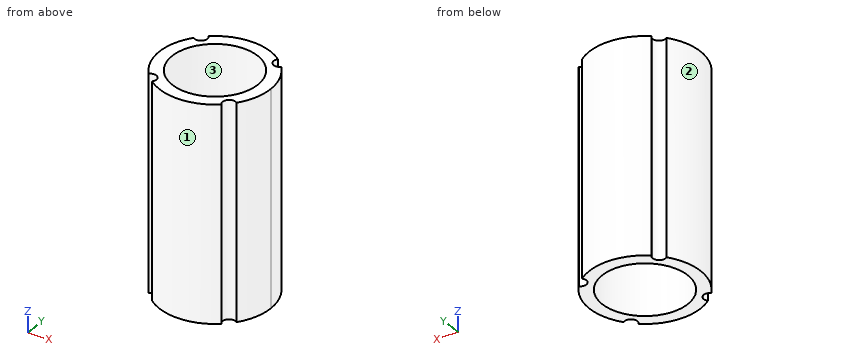
```python
from build123d import *

# Parameters (mm, degrees)
F0_R     = 12.7
F1_DEPTH = 63.5


with BuildPart() as f1:
    # F0 (on Top) → F1 (new body)
    with BuildSketch(Plane.XY):
        with BuildLine():
            ThreePointArc((12.941414, -10.251824), (15.592351, -5.427585), (16.51, 0))
            ThreePointArc((16.51, 0), (15.592351, 5.427585), (12.941414, 10.251824))
            ThreePointArc((12.941414, 10.251824), (10.327295, 10.327295), (10.251824, 12.941414))
            ThreePointArc((10.251824, 12.941414), (0, 16.51), (-10.251824, 12.941414))
            ThreePointArc((-10.251824, 12.941414), (-9.894038, 12.352251), (-9.769333, 11.674333))
            ThreePointArc((-9.769333, 11.674333), (-10.894835, 9.936113), (-12.941414, 10.251824))
            ThreePointArc((-12.941414, 10.251824), (-16.51, 0), (-12.941414, -10.251824))
            ThreePointArc((-12.941414, -10.251824), (-10.894835, -9.936113), (-9.769333, -11.674333))
            ThreePointArc((-9.769333, -11.674333), (-9.894038, -12.352251), (-10.251824, -12.941414))
            ThreePointArc((-10.251824, -12.941414), (0, -16.51), (10.251824, -12.941414))
            ThreePointArc((10.251824, -12.941414), (10.327295, -10.327295), (12.941414, -10.251824))
        make_face()
        Circle(F0_R, mode=Mode.SUBTRACT)
    extrude(amount=F1_DEPTH)


solid = f1.part
```
The model under review builds one solid part; all positions refer to its coordinate system, in mm. Face numbers are marked on the shaded views. Give positions to 0.01 mm unless a question says otherwise; leave off trailing zeros. Write each loop counter-clockwise with the first axis right and the second up, starting at its lowest first coordinate (ties: lowest second). Pieces come first, ordered by that corner, then holes. Notation, with made-up numbers: M 89.25,-30.75 L 95.25,-30.75 A17 cw 95.25,1.25 Z; hole C -32.5,36.5 d5. An arc over 180 degrees is marked long. Write item = value, one per line. Start each with the question number.
Q1. We need section B-B (z = 23.5). State the section outline as (x, y) points (3 decimals), plus the area to 3 significant figures.
Q2. We need section C-C (y = -3). State the section outline as (x, z) points, plus the area to 3 significant figures.
Q3. We need section A-A (x = 0). State the section outline as (y, z) points, plus the area to 3 significant figures.
Q4. Mouldability with a two-part tool opening along Y and no side actions: class the marked faces 1, 2 and 3 as released by +Y, released by -Y, zero draft, split by the parting line, or undercut.
Q5. Clearance check with flat-ended pins moving along their axes: pin 1 (4 mm diameter, centred on y = 3, z = 54.5, fed in from +X); pin 2 (6 mm diameter, centred on y = -10.5, z = 25, fed in from -X); pin 3 (1.5 mm diameter, centred on y = 10, z = 25, fed in from +X). State where each tip first meets the part, or that it passes through.
Q6. For line 1 (Y direction, x = 0, z = 33); line 2 (Y direction, x = -5, z = 18.5); line 3 (X direction, y = -10.5, z = 47.5), list the stretches that pass through material, from the lowest coordinate up.
Result set:
q1.outline = M -12.941,-10.252 A1.905 cw -9.769,-11.674 A1.905 cw -10.252,-12.941 A16.51 ccw 10.252,-12.941 A1.905 cw 12.941,-10.252 A16.51 ccw 16.51,0 A16.51 ccw 12.941,10.252 A1.905 cw 10.252,12.941 A16.51 ccw -10.252,12.941 A1.905 cw -9.769,11.674 A1.905 cw -12.941,10.252 A16.51 ccw Z; hole C 0,0 d25.4
q1.area = 327 mm2
q2.outline = M -16.24,0 L -12.34,0 L -12.34,63.5 L -16.24,63.5 Z; M 12.34,0 L 16.24,0 L 16.24,63.5 L 12.34,63.5 Z
q2.area = 495 mm2
q3.outline = M -16.51,0 L -12.7,0 L -12.7,63.5 L -16.51,63.5 Z; M 12.7,0 L 16.51,0 L 16.51,63.5 L 12.7,63.5 Z
q3.area = 484 mm2
q4.face_1 = released by -Y
q4.face_2 = split by the parting line
q4.face_3 = undercut
q5.pin_1 = 16.48
q5.pin_2 = -14.71
q5.pin_3 = 13.68
q6.line_1 = -16.51 to -12.7, 12.7 to 16.51
q6.line_2 = -15.73 to -11.67, 11.67 to 15.73
q6.line_3 = -10.17 to -7.14, 7.14 to 10.17
